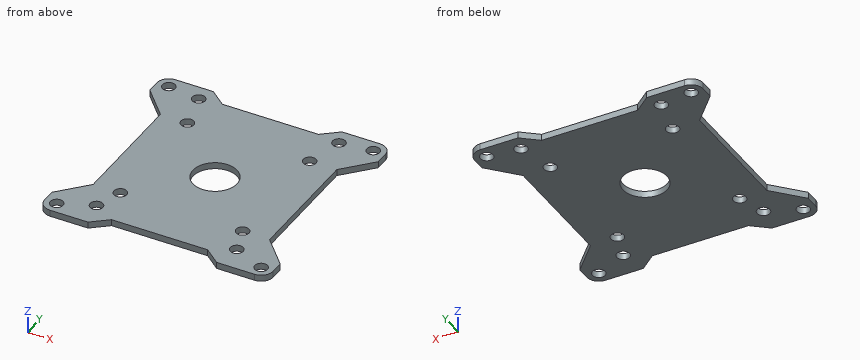
```python
from build123d import *

# Parameters (mm, degrees)
F0_R     = 1.6
F0_R_2   = 5.5
F1_DEPTH = 1.6


with BuildPart() as f1:
    # F0 (on Top) → F1 (new body)
    with BuildSketch(Plane.XY):
        with BuildLine():
            Line((-16.054926, 20.5), (-25.5, 20.5))
            ThreePointArc((-25.5, 20.5), (-27.62132, 19.62132), (-28.5, 17.5))
            Line((-28.5, 17.5), (-28.5, 14.321139))
            Line((-28.5, 14.321139), (-22.003273, 7.310869))
            Line((-22.003273, 7.310869), (-22.003273, -8))
            Line((-22.003273, -8), (-22.003273, -23.310869))
            Line((-22.003273, -23.310869), (-28.5, -30.321139))
            Line((-28.5, -30.321139), (-28.5, -33.5))
            ThreePointArc((-28.5, -33.5), (-27.62132, -35.62132), (-25.5, -36.5))
            Line((-25.5, -36.5), (-16.054926, -36.5))
            Line((-16.054926, -36.5), (-11.990136, -33.202917))
            Line((-11.990136, -33.202917), (0, -33.202917))
            Line((0, -33.202917), (11.990136, -33.202917))
            Line((11.990136, -33.202917), (16.054926, -36.5))
            Line((16.054926, -36.5), (25.5, -36.5))
            ThreePointArc((25.5, -36.5), (27.62132, -35.62132), (28.5, -33.5))
            Line((28.5, -33.5), (28.5, -30.321139))
            Line((28.5, -30.321139), (22.003273, -23.310869))
            Line((22.003273, -23.310869), (22.003273, -8))
            Line((22.003273, -8), (22.003273, 7.310869))
            Line((22.003273, 7.310869), (28.5, 14.321139))
            Line((28.5, 14.321139), (28.5, 17.5))
            ThreePointArc((28.5, 17.5), (27.62132, 19.62132), (25.5, 20.5))
            Line((25.5, 20.5), (16.054926, 20.5))
            Line((16.054926, 20.5), (11.990136, 17.202917))
            Line((11.990136, 17.202917), (0, 17.202917))
            Line((0, 17.202917), (-11.990136, 17.202917))
            Line((-11.990136, 17.202917), (-16.054926, 20.5))
        make_face()
        with Locations((-25.5, -33.5)):
            Circle(F0_R, mode=Mode.SUBTRACT)
        with Locations((-17.5, -30)):
            Circle(F0_R, mode=Mode.SUBTRACT)
        with Locations((-15.25, -23.25)):
            Circle(F0_R, mode=Mode.SUBTRACT)
        with Locations((17.5, -30)):
            Circle(F0_R, mode=Mode.SUBTRACT)
        with Locations((25.5, -33.5)):
            Circle(F0_R, mode=Mode.SUBTRACT)
        with Locations((15.25, -23.25)):
            Circle(F0_R, mode=Mode.SUBTRACT)
        with Locations((-15.25, 7.25)):
            Circle(F0_R, mode=Mode.SUBTRACT)
        with Locations((-25.5, 17.5)):
            Circle(F0_R, mode=Mode.SUBTRACT)
        with Locations((-17.500001, 16.5)):
            Circle(F0_R, mode=Mode.SUBTRACT)
        with Locations((0, -8)):
            Circle(F0_R_2, mode=Mode.SUBTRACT)
        with Locations((15.25, 7.25)):
            Circle(F0_R, mode=Mode.SUBTRACT)
        with Locations((17.500001, 16.5)):
            Circle(F0_R, mode=Mode.SUBTRACT)
        with Locations((25.5, 17.5)):
            Circle(F0_R, mode=Mode.SUBTRACT)
    extrude(amount=F1_DEPTH)


solid = f1.part
```
Verification items for the finished model (mm, model axes). Round coordinates to 2 decimals unless told otherwise and drop trailing zeros. Write each loop counter-clockwise with the first axis right and the second up, starting at its lowest first coordinate (ties: lowest second). Pieces come first, ordered by that corner, then holes.
1. Gauge pin test, flat ends, axial feed: P1, Ø0.8, axis at x = -1.5, z = 0.5, coming from the +Y side; P2, Ø3.5, axis at x = 15.25, y = -23.25, coming from the -Z side; P3, Ø3, axis at x = 25.5, y = 17.5, coming from the -Z side; P4, Ø0.5, axis at y = -15, z = 1, coming from the +X side. Record the tip position at first contact, or that the pin passes through.
2. Section check D-D on z = 0.5. State how many separate pieces and enclosed holes the cut face has, plus the area to 3 significant figures.
3. Section check B-B on y = -9. Enter the section's corners in (x, z).
4. Scan lines: L1, parallel to Y at x = -15.25, z = 1.2; L2, parallel to Y at x = -25, z = 0.3; L3, parallel to X at y = -24, z = 0.65. Record each from-to range of solid material in increasing order.
5. Section check A-A on x = 0. Enter the section's corners in (y, z).
6. Section check C-C on x = -15.25. Enter the section's corners in (y, z).
Answer:
1. P1: stops at y = 17.2
1. P2: stops at z = 0
1. P3: passes through
1. P4: stops at x = 22
2. separate pieces: 1
2. enclosed holes: 13
2. area: 2,380 mm2
3. outline: (-22, 0) - (-5.41, 0) - (-5.41, 1.6) - (-22, 1.6) - close; (5.41, 0) - (22, 0) - (22, 1.6) - (5.41, 1.6) - close
4. L1: y = -35.85 to -24.85, -21.65 to 5.65, 8.85 to 19.85
4. L2: y = -36.5 to -35.02, -31.98 to -26.54, 10.54 to 15.98, 19.02 to 20.5
4. L3: x = -22.64 to -16.66, -13.84 to 13.84, 16.66 to 22.64
5. outline: (-33.2, 0) - (-13.5, 0) - (-13.5, 1.6) - (-33.2, 1.6) - close; (-2.5, 0) - (17.2, 0) - (17.2, 1.6) - (-2.5, 1.6) - close
6. outline: (-35.85, 0) - (-24.85, 0) - (-24.85, 1.6) - (-35.85, 1.6) - close; (-21.65, 0) - (5.65, 0) - (5.65, 1.6) - (-21.65, 1.6) - close; (8.85, 0) - (19.85, 0) - (19.85, 1.6) - (8.85, 1.6) - close
